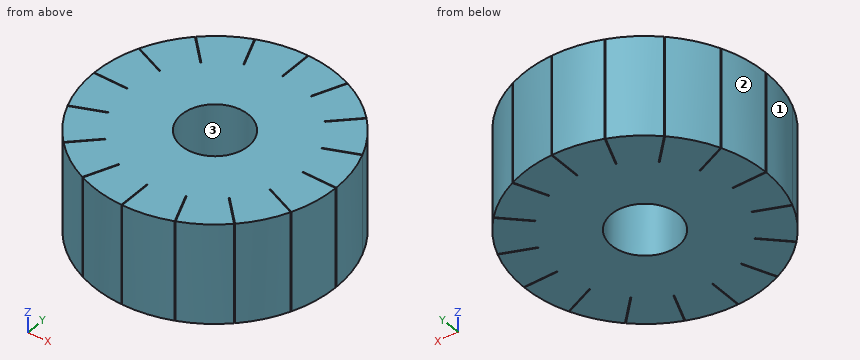
from build123d import *

# Parameters (mm, degrees)
ESQUISSE1_W                  = 12
ESQUISSE1_H                  = 10.5
ESQUISSE2_W                  = 0.1
ESQUISSE2_H                  = 4
ENL_V_MAT_EXTRU_2_DEPTH      = 24.759208741
R_P_TITION_CIRCULAIRE1_COUNT = 16


with BuildPart() as part:
    # Esquisse1 → R_volution1 (revolve)
    with BuildSketch(Plane(origin=(0, 0, 0), x_dir=(0, 0, -1), z_dir=(1, 0, 0)), mode=Mode.PRIVATE) as r_volution1_sk:
        with Locations((-6, 9.25)):
            Rectangle(ESQUISSE1_W, ESQUISSE1_H)
    revolve(r_volution1_sk.sketch.rotate(Axis((0, 0, 0), (0, 0, 1)), 90), axis=Axis((0, 0, 0), (0, 0, 1)))

    # Esquisse2 → Enl_v. mat.-Extru.2 (cut, through all)
    with BuildSketch(Plane.XY):
        with Locations((0, 12.5)):
            Rectangle(ESQUISSE2_W, ESQUISSE2_H)
    enl_v_mat_extru_2 = extrude(amount=ENL_V_MAT_EXTRU_2_DEPTH, mode=Mode.SUBTRACT)

    # R_p_tition circulaire1: Enl_v. mat.-Extru.2 ×16 about axis
    r_p_tition_circulaire1_axis = Axis((0, 0, 0), (0, 0, 1))
    for i in range(1, R_P_TITION_CIRCULAIRE1_COUNT):
        add(enl_v_mat_extru_2.rotate(r_p_tition_circulaire1_axis, i * 360 / R_P_TITION_CIRCULAIRE1_COUNT), mode=Mode.SUBTRACT)


solid = part.part
Geometry check sheet. Reference: the model listing, model coordinates, mm. Face numbers are marked on the shaded views. Give positions to 0.01 mm unless a question says otherwise; leave off trailing zeros. Loops run counter-clockwise (first coordinate to the right, second up) from the corner with the lowest first, then second, coordinate; pieces in that order, holes last. Notation, with made-up numbers: (-20, 39) -> (13, 39) arc R8 ccw to (13, 45) -> close; hole circle Ø2 at (-23.75, 76.25). An arc over 180 degrees is marked (long way). Answer in a Markdown table with one row per item. Add a question column.
1) Cross-section at A-A on y = -8.25. Record the boundary of the cut face in (x, z).
2) Cross-section at C-C on x = -6.5. Record the boundary of the cut face in (y, z).
3) Cross-section at B-B on x = 11.75. Record the boundary of the cut face in (y, z).
4) Material ranges on probe 1 along X at (y, z) = (-4.75, 2.75); probe 2 along Y at (x, z) = (0, 8.5); probe 3 along X at (y, z) = (-0.5, 7.25), recorded low to high. Write a range as from..to.
5) Draft check along Y on the marked faces 1, 2 and 3. Enter one of: pulls with the +Y half, pulls with the -Y half, needs draft (parallel to the pull), parting line crosses it, or undercut.
6) Gauge pin test, flat ends, axial feed: P1, Ø1.2, axis at x = -13, z = 6, coming from the +Y side; P2, Ø5, axis at y = -10.5, z = 5.5, coming from the -X side; P3, Ø5, axis at x = -3.5, z = 9, coming from the -Y side; P4, Ø5, axis at x = 11, y = 3.5, coming from the -Z side. Record the tip position at first contact, or that the pin passes through.
7) Cross-section at D-D on y = 6. Record the boundary of the cut face in (x, z).
Outcome:
| question | item | result |
|---|---|---|
| 1 | outline | (-11.92, 0) -> (-8.32, 0) -> (-8.32, 12) -> (-11.92, 12) -> close; (-8.18, 0) -> (8.18, 0) -> (8.18, 12) -> (-8.18, 12) -> close; (8.32, 0) -> (11.92, 0) -> (11.92, 12) -> (8.32, 12) -> close |
| 2 | outline | (-12.96, 0) -> (12.96, 0) -> (12.96, 12) -> (-12.96, 12) -> close |
| 3 | outline | (-8.5, 0) -> (-4.92, 0) -> (-4.92, 12) -> (-8.5, 12) -> close; (-4.81, 0) -> (-0.05, 0) -> (-0.05, 12) -> (-4.81, 12) -> close; (0.05, 0) -> (4.81, 0) -> (4.81, 12) -> (0.05, 12) -> close; (4.92, 0) -> (8.5, 0) -> (8.5, 12) -> (4.92, 12) -> close |
| 4 | probe 1 | x = -13.7..-11.6, -11.34..11.34, 11.6..13.7 |
| 4 | probe 2 | y = -10.5..-4, 4..10.5 |
| 4 | probe 3 | x = -14.49..-3.97, 3.97..14.49 |
| 5 | face 1 | pulls with the -Y half |
| 5 | face 2 | pulls with the +Y half |
| 5 | face 3 | undercut |
| 6 | P1 | stops at y = 7.52 |
| 6 | P2 | stops at x = -12.09 |
| 6 | P3 | stops at y = -14.47 |
| 6 | P4 | stops at z = 0 |
| 7 | outline | (-13.2, 0) -> (13.2, 0) -> (13.2, 12) -> (-13.2, 12) -> close |
